Input: part model. Units: mm. Frame: model coordinates. A direction names the side the tool comes from. Give positions to 0.01 mm unless a question says otherwise; leave off trailing zeros. Write each loop counter-clockwise with the first axis right and the second up, starting at its lowest first coordinate (ties: lowest second). Pieces come first, ordered by that corner, then holes. Notation, with made-up numbers: (71, 72) - (126, 72) arc R20 cw to (126, 106) - close; hole circle Ø6 at (-21, 85.5). An arc over 180 degrees is marked (long way). Use a Markdown table: item, result. Add a question column.
1. Material intervals for probe 1 along X at (y, z) = (23, 13.25); probe 2 along Y at (x, z) = (81.5, 16); probe 3 along X at (y, z) = (42, 16.75), sorted ascending.
2. Set-up query: faces 1 (the flat face through (20, 27, 15)), 2 (the cylindrical face through (114.293, 9.766, 1.774)), 3 (the flat face through (25, 13, 18)), 4 (the flat face through (0, 27, 2)), 5 (the flat face through (21, 41, 10)). Return all of +Z, -Z, +X, -X, +Y, -Y with unobstructed straight access to the full face (end or side cutting, diameter ignored); none if empty.
3. Section query B-B, the plane x = 76. Return loops of the section in (y, z).
4. Mould query, pull axis Z, two halves, no side actions, for faces 6 (the flat face through (62, 28, 6)), 7 (the flat face through (21, 35, 8.71)), 8 (the cylindrical face through (61.495, 42.721, 2.282)). Classes: released by +Z, released by -Z, zero draft, split by the parting line, or undercut.
5. Section query A-A, the plane z = 24. Return loops of the section in (x, y), plus the area to 3 significant figures.
6. Pin query (flat end, axial travel): pin 1 (1.8 mm diameter, centred on x = 115.79, y = 46, fed in from +Z); pin 2 (6 mm diameter, centred on x = 42.5, y = 14, fed in from +Z); pin 3 (2.5 mm diameter, centred on x = 101, y = 11, fed in from +Z); pin 4 (6 mm diameter, centred on x = 118, y = 38, fed in from +Z). Return the tip coordinate at first contact, or that it passes through.
```python
from build123d import *

# Parameters (mm, degrees)
F0_W      = 125
F0_H      = 55
F1_DEPTH  = 5
F2_W      = 85
F2_H      = 55
F3_DEPTH  = 21
F4_W      = 80.5
F4_H      = 36.3
F5_DEPTH  = 20
F6_R      = 2.5
F7_DEPTH  = 12
F8_W      = 12
F8_H      = 3
F9_DEPTH  = 25
F10_R     = 0.5
F11_DEPTH = 3
F12_R     = 1.5
F13_DEPTH = 25
F14_SIZE  = 1.5


with BuildPart() as f1:
    # F0 (on Top) → F1 (new body)
    with BuildSketch(Plane.XY):
        with Locations((62.5, 27.5)):
            Rectangle(F0_W, F0_H)
    extrude(amount=F1_DEPTH)

    # F2 (on face) → F3 (join)
    with BuildSketch(Plane.XY.offset(5)):
        with Locations((62.5, 27.5)):
            Rectangle(F2_W, F2_H)
    extrude(amount=F3_DEPTH)

    # F4 (on face) → F5 (cut)
    with BuildSketch(Plane.XY.offset(26)):
        with Locations((62.75, 27.85)):
            Rectangle(F4_W, F4_H)
    extrude(amount=-F5_DEPTH, mode=Mode.SUBTRACT)

    # F6 (on face) → F7 (join)
    with BuildSketch(Plane.XY.offset(6)):
        with Locations((25.5, 43)):
            Circle(F6_R)
        with Locations((100.4, 43.4)):
            Circle(F6_R)
        with Locations((100.4, 12.3)):
            Circle(F6_R)
        with Locations((25.5, 12.3)):
            Circle(F6_R)
    extrude(amount=F7_DEPTH)

    # F8 (on face) → F9 (cut)
    with BuildSketch(Plane(origin=(20, 0, 0), x_dir=(0, -1, 0), z_dir=(-1, 0, 0))):
        with Locations((-35, 10.209870059)):
            Rectangle(F8_W, F8_H)
    extrude(amount=-F9_DEPTH, mode=Mode.SUBTRACT)

    # F10 (on face) → F11 (cut)
    with BuildSketch(Plane.XY.offset(18)):
        with Locations((25.5, 43)):
            Circle(F10_R)
        with Locations((25.5017764866, 12)):
            Circle(F10_R)
        with Locations((100.5, 43.2148650289)):
            Circle(F10_R)
        with Locations((100.5017764866, 12.2148650289)):
            Circle(F10_R)
    extrude(amount=-F11_DEPTH, mode=Mode.SUBTRACT)

    # F12 (on face) → F13 (cut)
    with BuildSketch(Plane.XY.offset(6)):
        with Locations((62.6007243991, 41.7070947587)):
            Circle(F12_R)
        with Locations((63.5717511177, 14.8420426995)):
            Circle(F12_R)
        with Locations((6.820677314, 46)):
            Circle(F12_R)
        with Locations((6.820677314, 9.7)):
            Circle(F12_R)
        with Locations((115.7913729548, 46)):
            Circle(F12_R)
        with Locations((115.7913729548, 9.7)):
            Circle(F12_R)
    extrude(amount=-F13_DEPTH, mode=Mode.SUBTRACT)

    # F14
    f14_edges = [f1.edges().sort_by_distance(p)[0] for p in [
        (5.320677, 46, 5),
        (5.320677, 9.7, 5),
        (114.291373, 9.7, 5),
        (114.291373, 46, 5),
        (61.100724, 41.707095, 6),
        (62.071751, 14.842043, 6),
    ]]
    chamfer(f14_edges, length=F14_SIZE)


solid = f1.part
```
Result sheet:
| question | item | result |
|---|---|---|
| 1 | probe 1 | x = 20 to 22.5, 103 to 105 |
| 1 | probe 2 | y = 0 to 9.7, 46 to 55 |
| 1 | probe 3 | x = 20 to 22.5, 23.21 to 27.79, 98.33 to 102.47, 103 to 105 |
| 2 | face 1 | +Z, -X, +Y, -Y |
| 2 | face 2 | +Z, -Z |
| 2 | face 3 | +Z |
| 2 | face 4 | +Z, -Z, -X, +Y, -Y |
| 2 | face 5 | -X |
| 3 | outline | (0, 0) - (55, 0) - (55, 26) - (46, 26) - (46, 6) - (9.7, 6) - (9.7, 26) - (0, 26) - close |
| 4 | face 6 | released by +Z |
| 4 | face 7 | undercut |
| 4 | face 8 | zero draft |
| 5 | outline | (20, 0) - (105, 0) - (105, 55) - (20, 55) - close; hole (22.5, 9.7) - (103, 9.7) - (103, 46) - (22.5, 46) - close |
| 5 | area | 1,750 mm² |
| 6 | pin 1 | passes through |
| 6 | pin 2 | stops at z = 6 |
| 6 | pin 3 | stops at z = 18 |
| 6 | pin 4 | stops at z = 5 |
